```python
from build123d import *

# Parameters (mm, degrees)
SKETCH1_R               = 29.7
SKETCH1_R_2             = 20.8
BOSS_EXTRUDE1_DEPTH     = 6
SKETCH3_R               = 60
SKETCH3_R_2             = 29.7
BOSS_EXTRUDE2_DEPTH     = 15
CUT_EXTRUDE1_DEPTH      = 87.168439698
CUT_EXTRUDE1_DEPTH_BACK = 87.168439698
SKETCH4_R               = 3
CUT_EXTRUDE3_DEPTH      = 87.168439698
CUT_EXTRUDE3_DEPTH_BACK = 87.168439698
SKETCH2_R               = 2.5
SKETCH5_R               = 12.9
SKETCH5_R_2             = 3
BOSS_EXTRUDE3_DEPTH     = 2
CUT_EXTRUDE4_DEPTH      = 87.168439698
CUT_EXTRUDE4_DEPTH_BACK = 87.168439698
SKETCH5_2_R             = 3
CHAMFER1_SIZE           = 1


with BuildPart() as part:
    # Sketch1 → Boss-Extrude1 (new body)
    with BuildSketch(Plane.XY):
        Circle(SKETCH1_R)
        Circle(SKETCH1_R_2, mode=Mode.SUBTRACT)
    extrude(amount=BOSS_EXTRUDE1_DEPTH)

    # Sketch3 → Boss-Extrude2 (add)
    with BuildSketch(Plane.XY):
        with Locations(Location((0, 0, 0), (0, 0, 180))):
            Circle(SKETCH3_R)
        with Locations(Location((0, 0, 0), (0, 0, 180))):
            Circle(SKETCH3_R_2, mode=Mode.SUBTRACT)
    extrude(amount=BOSS_EXTRUDE2_DEPTH)

    # Sketch4 → Cut-Extrude1 (cut, two sides: drawn at the far end of the back side and taken through both)
    with BuildSketch(Plane.XY.offset(-CUT_EXTRUDE1_DEPTH_BACK)):
        with Locations(Location((-22.980970389, 22.980970389, 0), (0, 0, 294.931333751))):
            Circle(SKETCH4_R)
        with Locations(Location((22.980970389, 22.980970389, 0), (0, 0, 204.931333751))):
            Circle(SKETCH4_R)
        with Locations(Location((22.980970389, -22.980970389, 0), (0, 0, 155.068666249))):
            Circle(SKETCH4_R)
        with Locations(Location((-22.980970389, -22.980970389, 0), (0, 0, 65.068666249))):
            Circle(SKETCH4_R)
    extrude(amount=CUT_EXTRUDE1_DEPTH + CUT_EXTRUDE1_DEPTH_BACK, mode=Mode.SUBTRACT)

    # Sketch2 → Cut-Extrude3 (cut, two sides: drawn at the far end of the back side and taken through both)
    with BuildSketch(Plane.XY.offset(-CUT_EXTRUDE3_DEPTH_BACK)):
        with Locations((0, 24)):
            Circle(SKETCH2_R)
        with Locations((24, 0)):
            Circle(SKETCH2_R)
        with Locations((0, -24)):
            Circle(SKETCH2_R)
        with Locations((-24, 0)):
            Circle(SKETCH2_R)
    extrude(amount=CUT_EXTRUDE3_DEPTH + CUT_EXTRUDE3_DEPTH_BACK, mode=Mode.SUBTRACT)

    # Sketch5 → Boss-Extrude3 (add)
    # profile 1 of 2: a face of its own
    with BuildSketch(Plane.XY.offset(15)):
        with Locations((0, 45.9)):
            Circle(SKETCH5_R)
        with Locations((0, 45.9)):
            Circle(SKETCH5_R_2, mode=Mode.SUBTRACT)
    # profile 2 of 2: a face of its own
    with BuildSketch(Plane.XY.offset(15)):
        with Locations((0, -45.9)):
            Circle(SKETCH5_R)
        with Locations((0, -45.9)):
            Circle(SKETCH5_R_2, mode=Mode.SUBTRACT)
    extrude(amount=BOSS_EXTRUDE3_DEPTH)

    # Sketch5<2> → Cut-Extrude4 (cut, two sides: drawn at the far end of the back side and taken through both)
    with BuildSketch(Plane.XY.offset(15).offset(-CUT_EXTRUDE4_DEPTH_BACK)):
        with Locations((0, 45.9)):
            Circle(SKETCH5_2_R)
        with Locations((0, -45.9)):
            Circle(SKETCH5_2_R)
    extrude(amount=CUT_EXTRUDE4_DEPTH + CUT_EXTRUDE4_DEPTH_BACK, mode=Mode.SUBTRACT)

    # Chamfer1
    # the kernel refuses this chamfer: 1 mm, written as the material it takes off along each edge
    with BuildSketch(Plane(origin=(0, 0, 0), x_dir=(-1, 0, 0), z_dir=(0, 1, 0))) as chamfer1_piece_1:
        Polygon((60 - CHAMFER1_SIZE, 0), (60, CHAMFER1_SIZE), (60, 0), align=None)
    revolve(axis=Axis((0, 0, 0), (0, 0, 1)), mode=Mode.SUBTRACT)
    with BuildSketch(Plane(origin=(0, 0, 15), x_dir=(-1, 0, 0), z_dir=(0, 1, 0))) as chamfer1_piece_2:
        Polygon((60, -CHAMFER1_SIZE), (60 - CHAMFER1_SIZE, 0), (60, 0), align=None)
    revolve(axis=Axis((0, 0, 15), (0, 0, 1)), mode=Mode.SUBTRACT)
    with BuildSketch(Plane(origin=(0, 0, 15), x_dir=(0.742872020210988, 0.6694334631519742, 0), z_dir=(0.6694334631519742, -0.742872020210988, 0))) as chamfer1_piece_3:
        Polygon((29.7, -CHAMFER1_SIZE), (29.7 + CHAMFER1_SIZE, 0), (29.7, 0), align=None)
    revolve(axis=Axis((0, 0, 15), (0, 0, 1)), revolution_arc=95.953291469, mode=Mode.SUBTRACT)
    with BuildSketch(Plane(origin=(0, 0, 15), x_dir=(-0.6694334631519382, 0.7428720202110204, 0), z_dir=(0.7428720202110204, 0.6694334631519382, 0))) as chamfer1_piece_4:
        Polygon((29.7, -CHAMFER1_SIZE), (29.7 + CHAMFER1_SIZE, 0), (29.7, 0), align=None)
    revolve(axis=Axis((0, 0, 15), (0, 0, 1)), revolution_arc=95.953291469, mode=Mode.SUBTRACT)
    with BuildSketch(Plane(origin=(0, 0, 15), x_dir=(-0.7428720202113098, -0.6694334631516169, 0), z_dir=(-0.6694334631516169, 0.7428720202113098, 0))) as chamfer1_piece_5:
        Polygon((29.7, -CHAMFER1_SIZE), (29.7 + CHAMFER1_SIZE, 0), (29.7, 0), align=None)
    revolve(axis=Axis((0, 0, 15), (0, 0, 1)), revolution_arc=95.953291469, mode=Mode.SUBTRACT)
    with BuildSketch(Plane(origin=(0, 0, 15), x_dir=(0.6694334631516162, -0.7428720202113106, 0), z_dir=(-0.7428720202113106, -0.6694334631516162, 0))) as chamfer1_piece_6:
        Polygon((29.7, -CHAMFER1_SIZE), (29.7 + CHAMFER1_SIZE, 0), (29.7, 0), align=None)
    revolve(axis=Axis((0, 0, 15), (0, 0, 1)), revolution_arc=95.95329147, mode=Mode.SUBTRACT)
    with BuildSketch(Plane(origin=(0, 0, 0), x_dir=(1, 0, 0), z_dir=(0, -1, 0))) as chamfer1_piece_7:
        Polygon((20.8, CHAMFER1_SIZE), (20.8 + CHAMFER1_SIZE, 0), (20.8, 0), align=None)
    revolve(axis=Axis((0, 0, 0), (0, 0, 1)), mode=Mode.SUBTRACT)
    with BuildSketch(Plane(origin=(0, 0, 6), x_dir=(1, 0, 0), z_dir=(0, -1, 0))) as chamfer1_piece_8:
        Polygon((20.8, -CHAMFER1_SIZE), (20.8 + CHAMFER1_SIZE, 0), (20.8, 0), align=None)
    revolve(axis=Axis((0, 0, 6), (0, 0, 1)), mode=Mode.SUBTRACT)
    with BuildSketch(Plane(origin=(0, 45.9, 17), x_dir=(1, 0, 0), z_dir=(0, -1, 0))) as chamfer1_piece_9:
        Polygon((12.9, -CHAMFER1_SIZE), (12.9 - CHAMFER1_SIZE, 0), (12.9, 0), align=None)
    revolve(axis=Axis((0, 45.9, 17), (0, 0, 1)), mode=Mode.SUBTRACT)
    with BuildSketch(Plane(origin=(0, -45.9, 17), x_dir=(1, 0, 0), z_dir=(0, -1, 0))) as chamfer1_piece_10:
        Polygon((12.9, -CHAMFER1_SIZE), (12.9 - CHAMFER1_SIZE, 0), (12.9, 0), align=None)
    revolve(axis=Axis((0, -45.9, 17), (0, 0, 1)), mode=Mode.SUBTRACT)
    with BuildSketch(Plane(origin=(0, -45.9, 17), x_dir=(1, 0, 0), z_dir=(0, -1, 0))) as chamfer1_piece_11:
        Polygon((3, -CHAMFER1_SIZE), (3 + CHAMFER1_SIZE, 0), (3, 0), align=None)
    revolve(axis=Axis((0, -45.9, 17), (0, 0, 1)), mode=Mode.SUBTRACT)


solid = part.part
```
Design review of the part built by this model. Coordinates are the model's own, in mm. A direction names the side the tool comes from. Coordinates: 2 decimals unless noted, no trailing zeros. Answer in a Markdown table with one row per item.
(1) The part is to be moulded in two halves that separate along X. For faces 1 (the cylindrical face through (0.3, 29.7, 9.9)), 2 (the flat face through (2, 43, 17)), 3 (the cylindrical face through (-32.26, -50.59, 7.41)), say which applies: released by +X, released by -X, zero draft, split by the parting line, or undercut.
Checked values:
| item | result |
|---|---|
| face 1 | undercut |
| face 2 | zero draft |
| face 3 | split by the parting line |
(2) Clearance check with flat-ended pins moving along their axes: pin 1 (1.5 mm diameter, centred on y = 30.5, z = 6.5, fed in from -X); pin 2 (9.5 mm diameter, centred on x = -22.98, y = -22.98, fed in from +Z); pin 3 (10 mm diameter, centred on y = 21, z = 10, fed in from -X). State where each tip first meets the part, or that it passes through.
Checked values:
| item | result |
|---|---|
| pin 1 | x = -52.11 |
| pin 2 | z = 15 |
| pin 3 | x = -57.83 |
(3) Wall thickness on line 1 along Y through (x, z) = (0, 9.5); line 2 along Y through (x, z) = (-24, 2): over which ranges is each line inside the solid? List them lowest first. Write a range as from..to.
Checked values:
| item | result |
|---|---|
| line 1 | -60..-48.9, -42.9..-29.7, 29.7..42.9, 48.9..60 |
| line 2 | -54.99..-25.8, -20.16..-2.5, 2.5..20.16, 25.8..54.99 |
(4) For faces 4 (the cylindrical face through (-29.7, 0.3, 9.9)), 5 (the cylindrical face through (-2.708, 20.623, 2.972)), list the 3-axis set-ups (+Z, -Z, +X, -X, +Y, -Y) from which the entire face can be reached by the end or side of a thin tool; tool diameter is ignored.
Checked values:
| item | result |
|---|---|
| face 4 | +Z |
| face 5 | +Z, -Z |
